```python
from build123d import *

# Parameters (mm, degrees)
BOSS_EXTRUDE4_DEPTH  = 10
BOSS_EXTRUDE5_DEPTH  = 10
BOSS_EXTRUDE13_DEPTH = 10
SKETCH9_W            = 25
SKETCH9_H            = 20
BOSS_EXTRUDE14_DEPTH = 10
BOSS_EXTRUDE15_DEPTH = 10


with BuildPart() as part:
    # Sketch1 → Boss-Extrude4 (new body)
    with BuildSketch(Plane.XY):
        Polygon((-25, 0), (-25, 15), (-5, 15), (0, 5), (0, 0), align=None)
    extrude(amount=BOSS_EXTRUDE4_DEPTH)

    # Sketch3 → Boss-Extrude5 (add)
    with BuildSketch(Plane(origin=(0, 0, 0), x_dir=(-1, 0, 0), z_dir=(0, 0, -1))):
        Polygon((5, 15), (5, 0), (30, 0), (30, 5), (25, 15), align=None)
    extrude(amount=BOSS_EXTRUDE5_DEPTH)

    # Sketch4 → Boss-Extrude13 (add)
    with BuildSketch(Plane(origin=(0, 0, -10), x_dir=(-1, 0, 0), z_dir=(0, 0, -1))):
        Polygon((5, 15), (5, 25), (25, 25), (30, 20), (30, 15), align=None)
    extrude(amount=-BOSS_EXTRUDE13_DEPTH)

    # Sketch9 → Boss-Extrude14 (add)
    with BuildSketch(Plane(origin=(0, 0, -10), x_dir=(-1, 0, 0), z_dir=(0, 0, -1))):
        with Locations((17.5, 10)):
            Rectangle(SKETCH9_W, SKETCH9_H)
    extrude(amount=BOSS_EXTRUDE14_DEPTH)

    # Sketch10 → Boss-Extrude15 (add)
    with BuildSketch(Plane(origin=(0, 0, -10), x_dir=(-1, 0, 0), z_dir=(0, 0, -1))):
        Polygon((5, 20), (25, 25), (25, 20), align=None)
    extrude(amount=BOSS_EXTRUDE15_DEPTH)


solid = part.part
```
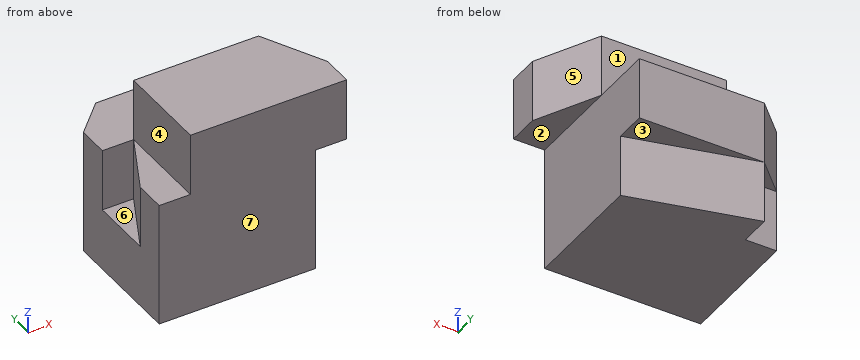
Model file for the job. Use its own axes, mm. Face numbers are marked on the shaded views. A direction names the side the tool comes from. Coordinates: 2 decimals unless noted, no trailing zeros. Loops run counter-clockwise (first coordinate to the right, second up) from the corner with the lowest first, then second, coordinate; pieces in that order, holes last. Notation, with made-up numbers: (61.25, -39.75) -> (77.25, -39.75) arc R24 ccw to (77.25, -17.75) -> close; hole circle Ø5 at (86.25, 82.5). An arc over 180 degrees is marked (long way). Answer as a JSON object with one key per item and string values.
Q1. 3-axis set-ups, long thin cutter, end or side, ignore diameter. For the marked faces 1, 2, 3 and 4: which of +Z, -Z, +X, -X, +Y, -Y reach the whole face in a straight line?
Report:
{"face 1": "+Z, +X, -X, +Y", "face 2": "-Z, +X, +Y, -Y", "face 3": "-Z, +X, +Y", "face 4": "+Z, -X, +Y, -Y"}
Q2. Cut at B-B (x = -20). List the corners of the cut face in (y, z).
Report:
{"outline": "(0, -20) -> (23.75, -20) -> (23.75, -10) -> (25, -10) -> (25, 0) -> (15, 0) -> (15, 10) -> (0, 10) -> close"}
Q3. Cut at C-C (z = -5.25). List the corners of the cut face in (x, y).
Report:
{"outline": "(-30, 0) -> (-5, 0) -> (-5, 25) -> (-25, 25) -> (-30, 20) -> (-30, 15) -> (-25, 15) -> (-30, 5) -> close"}
Q4. Flat gauge pins, fed straight in: P1, Ø4, axis at x = -28, y = 11.5, coming from the +Z side; P2, Ø5.5, axis at x = -1.5, y = 10.5, coming from the -Z side; P3, Ø10, axis at y = 10, z = -8.5, coming from the +X side. Where does each tip first touch, or does it go through?
Report:
{"P1": "stops at z = 0", "P2": "stops at z = 0", "P3": "stops at x = -5"}
Q5. Cut at D-D (z = -14.25). List the corners of the cut face in (x, y), and give its area (3 significant figures).
Report:
{"outline": "(-30, 0) -> (-5, 0) -> (-5, 20) -> (-25, 25) -> (-25, 20) -> (-30, 20) -> close", "area": "550 mm2"}
Q6. Cut at A-A (y = 6.5). List the corners of the cut face in (x, z).
Report:
{"outline": "(-30, -20) -> (-5, -20) -> (-5, 0) -> (-0.75, 0) -> (-0.75, 10) -> (-25, 10) -> (-25, 0) -> (-29.25, 0) -> (-29.25, -10) -> (-30, -10) -> close"}
Q7. Pull direction Y, two halves, no side cores. Call the marked faces 5, 6 and 7: released by +Y, released by -Y, zero draft, split by the parting line, or undercut.
Report:
{"face 5": "released by +Y", "face 6": "undercut", "face 7": "released by -Y"}
Q8. Probe probe 1 along Z at (x, y) = (-26.5, 17.25); probe 2 along Y at (x, z) = (-7.5, 6); probe 3 along X at (y, z) = (15.25, -11.25). List the from-to ranges inside material, lowest first.
Report:
{"probe 1": "z = -20 to 0", "probe 2": "y = 0 to 15", "probe 3": "x = -30 to -5"}
